Geometry check sheet. Reference: the model listing, model coordinates, mm. A direction names the side the tool comes from. Give positions to 0.01 mm unless a question says otherwise; leave off trailing zeros. Write each loop counter-clockwise with the first axis right and the second up, starting at its lowest first coordinate (ties: lowest second). Pieces come first, ordered by that corner, then holes. Notation, with made-up numbers: M 89,77.25 L 106,77.25 A14 ccw 106,93.25 Z; hole C 86.5,38 d11. An arc over 180 degrees is marked long. Write each question's results on one line, items separated by ' | '.
```python
from build123d import *

# Parameters (mm, degrees)
SKETCH_1_R      = 3.175
EXTRUDE_1_DEPTH = 88.9


with BuildPart() as part:
    # Эскиз1 → Бобышка-Вытянуть1 (new body)
    with BuildSketch(Plane(origin=(0, 0, 0), x_dir=(1, 0, 0), z_dir=(0, 1, 0))):
        with BuildLine():
            Line((-194.590147989, 18.24646839), (-194.590147989, -19.85353161))
            Line((-194.590147989, -19.85353161), (-155.294835417, -19.85353161))
            ThreePointArc((-155.294835417, -19.85353161), (-140.960808265, -67.827276327), (-111.853221442, -108.566605063))
            ThreePointArc((-111.853221442, -108.566605063), (-71.113892706, -137.674191886), (-23.140147989, -152.008219038))
            Line((-23.140147989, -152.008219038), (-23.140147989, -191.30353161))
            Line((-23.140147989, -191.30353161), (14.959852011, -191.30353161))
            Line((14.959852011, -191.30353161), (14.959852011, -152.008219038))
            ThreePointArc((14.959852011, -152.008219038), (62.933596727, -137.674191886), (103.672925464, -108.566605063))
            ThreePointArc((103.672925464, -108.566605063), (132.780512286, -67.827276327), (147.114539438, -19.85353161))
            Line((147.114539438, -19.85353161), (186.409852011, -19.85353161))
            Line((186.409852011, -19.85353161), (186.409852011, 18.24646839))
            Line((186.409852011, 18.24646839), (147.114539438, 18.24646839))
            ThreePointArc((147.114539438, 18.24646839), (132.780512286, 66.220213106), (103.672925464, 106.959541842))
            ThreePointArc((103.672925464, 106.959541842), (62.933596727, 136.067128665), (14.959852011, 150.401155817))
            Line((14.959852011, 150.401155817), (14.959852011, 189.69646839))
            Line((14.959852011, 189.69646839), (-23.140147989, 189.69646839))
            Line((-23.140147989, 189.69646839), (-23.140147989, 150.401155817))
            ThreePointArc((-23.140147989, 150.401155817), (-71.113892706, 136.067128665), (-111.853221442, 106.959541842))
            ThreePointArc((-111.853221442, 106.959541842), (-140.960808265, 66.220213106), (-155.294835417, 18.24646839))
            Line((-155.294835417, 18.24646839), (-194.590147989, 18.24646839))
        make_face()
        with Locations(Location((-175.540147989, -0.80353161, 0), (0, 0, 270))):
            Circle(SKETCH_1_R, mode=Mode.SUBTRACT)
        with Locations(Location((-99.340147989, 0, 0), (0, 0, 90))):
            Circle(SKETCH_1_R, mode=Mode.SUBTRACT)
        with Locations(Location((-4.090147989, 170.64646839, 0), (0, 0, 270))):
            Circle(SKETCH_1_R, mode=Mode.SUBTRACT)
        with Locations(Location((-3.286616379, 94.44646839, 0), (0, 0, 90))):
            Circle(SKETCH_1_R, mode=Mode.SUBTRACT)
        with Locations(Location((167.359852011, -0.80353161, 0), (0, 0, 270))):
            Circle(SKETCH_1_R, mode=Mode.SUBTRACT)
        with Locations(Location((91.159852011, -1.607063221, 0), (0, 0, 90))):
            Circle(SKETCH_1_R, mode=Mode.SUBTRACT)
        with Locations(Location((-4.090147989, -172.25353161, 0), (0, 0, 270))):
            Circle(SKETCH_1_R, mode=Mode.SUBTRACT)
        with Locations(Location((-4.8936796, -96.05353161, 0), (0, 0, 90))):
            Circle(SKETCH_1_R, mode=Mode.SUBTRACT)
        with BuildLine():
            Line((-77.870480735, 18.24646839), (-116.791467857, 18.24646839))
            ThreePointArc((-116.791467857, 18.24646839), (-84.912453079, 80.018773479), (-23.140147989, 111.897788258))
            Line((-23.140147989, 111.897788258), (-23.140147989, 72.976801135))
            ThreePointArc((-23.140147989, 72.976801135), (-4.090147989, 75.39646839), (14.959852011, 72.976801135))
            Line((14.959852011, 72.976801135), (14.959852011, 111.897788258))
            ThreePointArc((14.959852011, 111.897788258), (76.7321571, 80.018773479), (108.611171879, 18.24646839))
            Line((108.611171879, 18.24646839), (69.690184756, 18.24646839))
            ThreePointArc((69.690184756, 18.24646839), (72.109852011, -0.80353161), (69.690184756, -19.85353161))
            Line((69.690184756, -19.85353161), (108.611171879, -19.85353161))
            ThreePointArc((108.611171879, -19.85353161), (76.7321571, -81.6258367), (14.959852011, -113.504851478))
            Line((14.959852011, -113.504851478), (14.959852011, -74.583864356))
            ThreePointArc((14.959852011, -74.583864356), (-4.090147989, -77.00353161), (-23.140147989, -74.583864356))
            Line((-23.140147989, -74.583864356), (-23.140147989, -113.504851478))
            ThreePointArc((-23.140147989, -113.504851478), (-84.912453079, -81.6258367), (-116.791467857, -19.85353161))
            Line((-116.791467857, -19.85353161), (-77.870480735, -19.85353161))
            ThreePointArc((-77.870480735, -19.85353161), (-80.290147989, -0.80353161), (-77.870480735, 18.24646839))
        make_face(mode=Mode.SUBTRACT)
    extrude(amount=EXTRUDE_1_DEPTH)


solid = part.part
```
Q1. Section check D-D (x = 115). Enter the section's corners in (y, z), then the cut area to 3 significant figures.
Answer key:
outline: M 0,-94.29 L 88.9,-94.29 L 88.9,95.9 L 0,95.9 Z | area: 16,900 mm2
Q2. Section check A-A (z = 40). Enter the section's corners in (x, y), then the cut area to 3 significant figures.
Answer key:
outline: M -151.36,0 L -111.46,0 L -111.46,88.9 L -151.36,88.9 Z; M 103.28,0 L 143.18,0 L 143.18,88.9 L 103.28,88.9 Z | area: 7,090 mm2
Q3. Section check C-C (y = 61.5). State how many separate pieces and enclosed holes the cut face has, then the cut area to 3 significant figures.
Answer key:
separate pieces: 1 | enclosed holes: 9 | area: 43,400 mm2
Q4. Material ranges on probe 1 along Z at (x, y) = (-5.5, 15.5); probe 2 along Z at (x, y) = (99.5, 76.5); probe 3 along Z at (x, y) = (-93, 69.5), recorded low to high. Write a range as [from, to].
Answer key:
probe 1: z = [-189.7, -173.49], [-167.8, -96.72], [-92.17, -75.38], [76.99, 92.94], [99.17, 169.41], [175.1, 191.3] | probe 2: z = [-110.98, -47.5], [-18.25, 19.85], [49.11, 112.58] | probe 3: z = [-122.97, -71.03], [-18.25, 19.85], [72.63, 124.58]
Q5. Access from +Z, -Z, +X, -X, +Y, -Y to the whole of each face (thin tool, end or side, straight path). Record for faces 4 (the face through (14.96, 44, -170)), 5 (the face through (-23.14, 44, -170)), 6 (the face through (166, 44, 19.854)), 7 (the face through (-80.29, 43.83, 1.07)), 8 (the face through (-19, 0, -85)).
Answer key:
face 4: -Z, +X, +Y, -Y | face 5: -Z, -X, +Y, -Y | face 6: +Z, +X, +Y, -Y | face 7: +Y, -Y | face 8: +Z, -Z, +X, -X, -Y
Q6. Section check B-B (x = -61.5). Enter the section's corners in (y, z).
Answer key:
outline: M 0,-140.37 L 88.9,-140.37 L 88.9,-98.03 L 0,-98.03 Z; M 0,99.64 L 88.9,99.64 L 88.9,141.98 L 0,141.98 Z
Q7. Release check for a two-part mould opening along X. For faces 1 (the face through (-23.14, 44, 171)), 2 (the face through (104.664, 43.828, -105.959)), 3 (the face through (14.96, 44, -92)) record: released by +X, released by -X, zero draft, split by the parting line, or undercut.
Answer key:
face 1: released by -X | face 2: released by +X | face 3: undercut
Q8. Depth check by flat-ended pin: P1, Ø12, axis at x = 167, y = 28.5, coming from the +Z side; P2, Ø8, axis at y = 66, z = 77, coming from the -X side; P3, Ø19.5, axis at y = 49.5, z = -89.5, coming from the -X side; P4, Ø4, axis at x = -3.29, z = -94.45, coming from the +Y side. Enter the tip coordinate at first touch or a pass-through.
Answer key:
P1: stops at z = 19.85 | P2: stops at x = -138.3 | P3: stops at x = -133.46 | P4: passes through
